```python
from build123d import *

# Parameters (mm, degrees)
SKETCH1_R              = 12.7
SKETCH1_R_2            = 2.0193
BOSS_EXTRUDE1_DEPTH    = 82.2325
F_10_32_TAPPED_HOLE1_D = 4.0386
F_10_32_TAPPED_HOLE2_D = 4.0386


with BuildPart() as part:
    # Sketch1 → Boss-Extrude1 (new body)
    with BuildSketch(Plane.XY):
        Circle(SKETCH1_R)
        Circle(SKETCH1_R_2, mode=Mode.SUBTRACT)
    extrude(amount=BOSS_EXTRUDE1_DEPTH)

    # #10-32 Tapped Hole1 (through all)
    with Locations(Plane.XY.offset(82.2325)):
        with Locations((0, 0)):
            Hole(F_10_32_TAPPED_HOLE1_D / 2)

    # #10-32 Tapped Hole2 (through all)
    with Locations(Plane(origin=(0, 0, 0), x_dir=(-1, 0, 0), z_dir=(0, 0, -1))):
        with Locations((0, 0)):
            Hole(F_10_32_TAPPED_HOLE2_D / 2)


solid = part.part
```
Model file for the job. Use its own axes, mm. Round coordinates to 2 decimals unless told otherwise and drop trailing zeros. Write each loop counter-clockwise with the first axis right and the second up, starting at its lowest first coordinate (ties: lowest second). Pieces come first, ordered by that corner, then holes. Notation, with made-up numbers: (84.5, 49.25) - (141.5, 49.25) arc R19 cw to (141.5, 85.25) - close; hole circle Ø5 at (-10.5, -12). An arc over 180 degrees is marked (long way). One line per item, written item: value.
(1) Drop flat-ended pins along their axis: P1, Ø4, axis at x = -8, z = 53.5, coming from the +Y side; P2, Ø3, axis at x = 10, z = 14, coming from the +Y side; P3, Ø4, axis at x = 8.5, y = 9, coming from the -Z side; P4, Ø5, axis at y = -5, z = 18, coming from the -X side. Give the stop position or say it passes through.
Values follow:
P1: stops at y = 11.19
P2: stops at y = 9.44
P3: stops at z = 0
P4: stops at x = -12.45
(2) Wall check: probe 1 along Y at (x, z) = (0, 48); probe 2 along Y at (x, z) = (-9.75, 77); probe 3 along Y at (x, z) = (9.25, 46.5). Give the ranges that are in metal, low to high.
Values follow:
probe 1: y = -12.7 to -2.02, 2.02 to 12.7
probe 2: y = -8.14 to 8.14
probe 3: y = -8.7 to 8.7
(3) Cut at C-C, the plane z = 69.5. Give the cut face in (x, y).
Values follow:
outline: circle Ø25.4 at (0, 0); hole circle Ø4.04 at (0, 0)
(4) Cut at D-D, the plane y = -3.75. Give the cut face in (x, z), plus the area to 3 significant figures.
Values follow:
outline: (-12.13, 0) - (12.13, 0) - (12.13, 82.23) - (-12.13, 82.23) - close
area: 2,000 mm²
(5) Two-plate mould, pull along Y, no slides. Class faces 1 (the flat face through (3, 0, 82.232)), 2 (the cylindrical face through (-2.75, -12.4, 40.54)), 3 (the cylindrical face through (1.926, 0.607, 40.541)): pulls with the +Y half, pulls with the -Y half, needs draft (parallel to the pull), parting line crosses it, or undercut.
Values follow:
face 1: needs draft
face 2: parting line crosses it
face 3: undercut
(6) Cut at A-A, the plane y = 0. Give the cut face in (x, z).
Values follow:
outline: (-12.7, 0) - (-2.02, 0) - (-2.02, 82.23) - (-12.7, 82.23) - close; (2.02, 0) - (12.7, 0) - (12.7, 82.23) - (2.02, 82.23) - close
